Could you check a few things on this model? Use its own coordinates, in mm. Face numbers are marked on the shaded views. Give positions to 0.01 mm unless a question says otherwise; leave off trailing zeros. Loops run counter-clockwise (first coordinate to the right, second up) from the corner with the lowest first, then second, coordinate; pieces in that order, holes last.
1. I need wall thicknesses on line 1 along Z through (x, y) = (11, 5.75); line 2 along X through (y, z) = (7, -31); line 3 along Z through (x, y) = (9, 17.75). Which ranges of each line are inside material? Lowest first, please.
2. Imagine slicing it at D-D (y = 17). Count the separate pieces of the cut face and the enclosed holes in it, plus the area to 3 significant figures.
3. Imagine slicing it at C-C (z = -31.5). List the corners of the cut face in (x, y) for me.
4. Imagine slicing it at B-B (z = -11.4). List the corners of the cut face in (x, y) for me.
5. Thinking about a two-plate mould opening in X: for the marked faces 1, 2, 3 and 4, which applies, +X half, -X half, draft (parallel to the pull), parting line (faces both ways), or undercut?
6. For P1, Ø5, axis at x = 12.5, y = 7.5, coming from the +Z side; P2, Ø4, axis at y = 7, z = -42, coming from the -X side, each with a flat end and sliding along its axis, tell me the tip position at first contact or that it passes through.
7. Imagine slicing it at A-A (x = 11). List the corners of the cut face in (y, z) for me, plus the area to 3 significant figures.
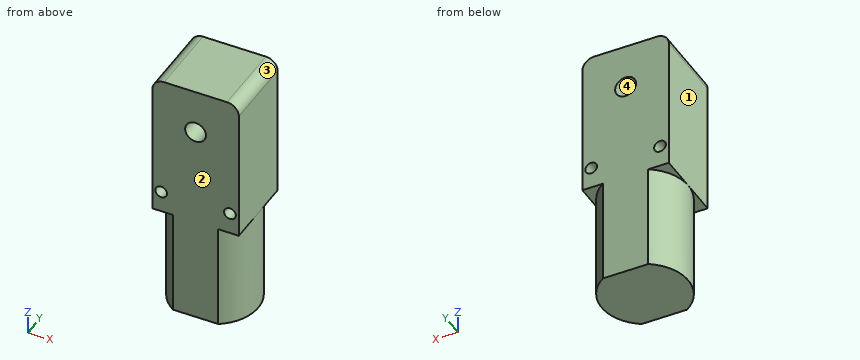
Autodesk Inventor part; units mm, degrees
ref_plane "YZ Plane" through (0, 0, 0) normal (1, 0, 0) x (0, 1, 0)
ref_plane "XZ Plane" through (0, 0, 0) normal (0, 1, 0) x (-1, 0, 0)
ref_plane "XY Plane" through (0, 0, 0) normal (0, 0, 1) x (1, 0, 0)
sketch "Sketch1" plane through (0, 0, 0) normal (0, 1, 0) x (-1, 0, 0)
  line L0 (0, 0) -> (-22, 0)
  line L1 (-22, 0) -> (-22, -37)
  line L2 (-22, -37) -> (0, -37)
  line L3 (0, -37) -> (0, 0)
  line L4 (-11, -37) -> (-11, 0) construction
  circle A0 centre (-11, -11.4) radius 2.65
  circle A1 centre (-19.75, -31.5) radius 1.5
  circle A2 centre (-2.25, -31.5) radius 1.5
  dimension "gearboxWidth" = 22
  dimension "gearboxLength" = 37
  dimension "shaftDiameter" = 5.3
  dimension "shaftCenterToBottom" = 11.4
  dimension "mountHolesDiameter" = 3
  dimension "mountHolesCenterToCenter" = 17.5
  dimension "mountHolesCenterToEdge" = 5.5
extrude "Extrusion1" add sketch "Sketch1" along normal blind 19
sketch "Sketch2" plane through (22, 0, -37) normal (0, 0, -1) x (-1, 0, 0)
  line L0 (0, 19) -> (22, 19)
  line L1 (11, 19) -> (11, 0) construction
  line L2 (0, 0) -> (22, 0)
  ellipse E0 centre (11, 9.5) end of major axis (22, 9.5) minor radius 11.1399 (16.7448, 0) -> (16.7448, 19) ccw
  ellipse E1 centre (11, 9.5) end of major axis (22, 9.5) minor radius 11.1399 (5.2552, 19) -> (5.2552, 0) ccw
  line L3 (5.2552, 19) -> (16.7448, 19)
  line L4 (5.2552, 0) -> (16.7448, 0)
extrude "Extrusion2" add sketch "Sketch2" along normal blind 27
fillet "Fillet1" radius 3 2 edges at (0, 9.5, 0) (22, 9.5, 0)
properties part number "Yellow_Motor"
Derived:
1. line 1: z = -64 to -14.05, -8.75 to 0
1. line 2: x = 0 to 0.84, 3.66 to 18.34, 21.16 to 22
1. line 3: z = -64 to -13.14, -9.66 to 0
2. separate pieces: 1
2. enclosed holes: 3
2. area: 1,210 mm2
3. outline: (0, 0) - (0.75, 0) - (0.75, 19) - (0, 19) - close; (3.75, 0) - (18.25, 0) - (18.25, 19) - (3.75, 19) - close; (21.25, 0) - (22, 0) - (22, 19) - (21.25, 19) - close
4. outline: (0, 0) - (8.35, 0) - (8.35, 19) - (0, 19) - close; (13.65, 0) - (22, 0) - (22, 19) - (13.65, 19) - close
5. face 1: -X half
5. face 2: draft
5. face 3: +X half
5. face 4: undercut
6. P1: stops at z = 0
6. P2: stops at x = 0.01
7. outline: (0, -64) - (19, -64) - (19, -14.05) - (0, -14.05) - close; (0, -8.75) - (19, -8.75) - (19, 0) - (0, 0) - close
7. area: 1,120 mm2
